```python
from build123d import *

# Parameters (mm, degrees)
CROQUIS2_OUTSIDE_W    = 65.964
CROQUIS2_OUTSIDE_H    = 65.964
CROQUIS2_OUTSIDE_W_2  = 60
CROQUIS2_OUTSIDE_H_2  = 40
CORTAR_EXTRUIR1_DEPTH = 10


with BuildPart() as part:
    # Croquis1 → Revolución1 (revolve)
    with BuildSketch(Plane.XY, mode=Mode.PRIVATE) as revoluci_n1_sk:
        Polygon((0, 8), (0, 24), (-10, 24), (-10, 14), (-42, 14), (-42, 8), align=None)
    revolve(revoluci_n1_sk.sketch.rotate(Axis((0, 0, 0), (-1, 0, 0)), 90), axis=Axis((0, 0, 0), (-1, 0, 0)))

    # Croquis2 outside → Cortar-Extruir1 (cut)
    with BuildSketch(Plane(origin=(0, 0, 0), x_dir=(0, 0, -1), z_dir=(1, 0, 0))):
        Rectangle(CROQUIS2_OUTSIDE_W, CROQUIS2_OUTSIDE_H)
        Rectangle(CROQUIS2_OUTSIDE_W_2, CROQUIS2_OUTSIDE_H_2, mode=Mode.SUBTRACT)
    extrude(amount=-CORTAR_EXTRUIR1_DEPTH, mode=Mode.SUBTRACT)


solid = part.part
```
Can you work these out from the model? Positions are in its coordinate system, mm. A direction names the side the tool comes from. Coordinates: 2 decimals unless noted, no trailing zeros. Order: outer loops, then holes, each group sorted by start corner. A loop starts at its lowest first (then second) coordinate and runs counter-clockwise, first axis right, second up. Notation, with made-up numbers: (88, 80) -> (133, 80) arc R14 ccw to (133, 96) -> close; hole circle Ø9 at (53, 59). An arc over 180 degrees is marked (long way). Write each question's results on one line, items separated by ' | '.
Item 1: I'm going to push flat-ended pins straight in: pin 1 Ø2 at (x, y) = (-10.5, 1) entering from +Z; pin 2 Ø1 at (x, y) = (-31.5, -12) entering from +Z; pin 3 Ø8 at (y, z) = (-11, 10.5) entering from -X; pin 4 Ø12 at (x, y) = (-31, 11.5) entering from +Z. Where does each tip first touch, or does it pass through?
Results are:
pin 1: z = 24 | pin 2: z = 7.98 | pin 3: x = -42 | pin 4: z = 12.87
Item 2: If I drill on line 1 along Y through (x, z) = (-21.5, 0); line 2 along Y through (x, z) = (-3, 19.5); line 3 along X through (y, z) = (-4, 14.5), over which ranges is the centre line in solid material (lowest first)?
Results are:
line 1: -14 to -8, 8 to 14 | line 2: -13.99 to 13.99 | line 3: -10 to 0
Item 3: I want a section at C-C, the plane x = -20.5. Write out the boundary of the cut face in (y, z).
Results are:
outline: circle Ø28 at (0, 0); hole circle Ø16 at (0, 0)
Item 4: I want a section at D-D, the plane y = 10. Write out the boundary of the cut face in (x, z), then the cut area to 3 significant figures.
Results are:
outline: (-42, -9.8) -> (-10, -9.8) -> (-10, -21.82) -> (0, -21.82) -> (0, 21.82) -> (-10, 21.82) -> (-10, 9.8) -> (-42, 9.8) -> close | area: 1,060 mm²
Item 5: Which directions (+Z, -Z, +X, -X, +Y, -Y) give clear straight access to the entire face, cutting with the end or side of a thin tool? Please do faces 1 (the face through (-20.71, 7.81, 1.73)), 2 (the face through (-10, -9, 11)).
Results are:
face 1: +X, -X | face 2: -X
Item 6: I want a section at A-A, the plane y = 0. Write out the boundary of the cut face in (x, z).
Results are:
outline: (-42, -14) -> (-10, -14) -> (-10, -24) -> (0, -24) -> (0, -8) -> (-42, -8) -> close; (-42, 8) -> (0, 8) -> (0, 24) -> (-10, 24) -> (-10, 14) -> (-42, 14) -> close
Item 7: I want a section at B-B, the plane z = 0. Write out the boundary of the cut face in (x, y), then the cut area to 3 significant figures.
Results are:
outline: (-42, -14) -> (-10, -14) -> (-10, -20) -> (0, -20) -> (0, -8) -> (-42, -8) -> close; (-42, 8) -> (0, 8) -> (0, 20) -> (-10, 20) -> (-10, 14) -> (-42, 14) -> close | area: 624 mm²
